Check sheet for the modelled part. Datum: model origin and axes. Units: mm. A direction names the side the tool comes from. Give positions to 0.01 mm unless a question says otherwise; leave off trailing zeros. Write each loop counter-clockwise with the first axis right and the second up, starting at its lowest first coordinate (ties: lowest second). Pieces come first, ordered by that corner, then holes. Notation, with made-up numbers: (-5.75, 47.25) -> (15.25, 47.25) arc R26 cw to (15.25, 74.25) -> close; hole circle Ø1 at (62, -2). An arc over 180 degrees is marked (long way). Write each question's results on one line, items separated by ' | '. Start each with the question number.
```python
from build123d import *

# Parameters (mm, degrees)
F0_W     = 74.9129392207
F0_H     = 89.2662387341
F0_H_2   = 11.6326007992
F1_DEPTH = 25.4
F3_DEPTH = 38.1
F4_W     = 74.9129392207
F4_H     = 18.2247254997
F5_DEPTH = 76.2
F7_DEPTH = 25.4
F8_W     = 15.1206124574
F8_H     = 39.1616150737
F9_DEPTH = 38.1


with BuildPart() as f1:
    # F0 (on Front) → F1 (new body)
    with BuildSketch(Plane.XZ):
        with Locations((-0.0017788261, 17.1041050926)):
            Rectangle(F0_W, F0_H)
        with Locations((-0.0017788261, -33.3453146741)):
            Rectangle(F0_W, F0_H_2)
    extrude(amount=F1_DEPTH)

    # F2 (on face) → F3 (cut, symmetric)
    with BuildSketch(Plane.XZ.offset(25.4)):
        with BuildLine():
            Line((8.0494598543, 36.3066755235), (8.2423314452, 36.3066755235))
            Line((8.2423314452, 36.3066755235), (8.2423314452, 87.1677733958))
            Line((8.2423314452, 87.1677733958), (-8.2423314452, 87.1677733958))
            Line((-8.2423314452, 87.1677733958), (-8.2423314452, 36.3066755235))
            Line((-8.2423314452, 36.3066755235), (-8.0494598543, 36.3066755235))
            ThreePointArc((-8.0494598543, 36.3066755235), (0, 44.3561353778), (8.0494598543, 36.3066755235))
        make_face()
        with BuildLine():
            ThreePointArc((-8.0494598543, 36.3066755235), (0, 28.2572156693), (8.0494598543, 36.3066755235))
            Line((8.0494598543, 36.3066755235), (-8.0494598543, 36.3066755235))
        make_face()
        with BuildLine():
            Line((-8.0494598543, 36.3066755235), (8.0494598543, 36.3066755235))
            ThreePointArc((8.0494598543, 36.3066755235), (0, 44.3561353778), (-8.0494598543, 36.3066755235))
        make_face()
    extrude(amount=F3_DEPTH, both=True, mode=Mode.SUBTRACT)

    # F4 (on face) → F5 (join)
    with BuildSketch(Plane.XZ.offset(25.4)):
        with Locations((-0.0017788261, -30.0492523238)):
            Rectangle(F4_W, F4_H)
    extrude(amount=F5_DEPTH)

    # F6 (on face) → F7 (cut)
    with BuildSketch(Plane.XY.offset(-20.9368895739)):
        with BuildLine():
            ThreePointArc((2.131e-07, -101.6), (-24.3546974871, -92.7994660414), (-37.4582484365, -70.4634491506))
            Line((-37.4582484365, -70.4634491506), (-37.4582484365, -101.6))
            Line((-37.4582484365, -101.6), (2.131e-07, -101.6))
        make_face()
        with BuildLine():
            ThreePointArc((37.4546907842, -70.4825595779), (24.3472225116, -92.8056778794), (2.131e-07, -101.6))
            Line((2.131e-07, -101.6), (37.4546907842, -101.6))
            Line((37.4546907842, -101.6), (37.4546907842, -70.4825595779))
        make_face()
    extrude(amount=-F7_DEPTH, mode=Mode.SUBTRACT)

    # F8 (on face) → F9 (cut)
    with BuildSketch(Plane(origin=(0, 0, 0), x_dir=(-1, 0, 0), z_dir=(0, 1, 0))):
        with Locations((-29.8943845555, -19.5808075368)):
            Rectangle(F8_W, F8_H)
    extrude(amount=-F9_DEPTH, mode=Mode.SUBTRACT)


solid = f1.part
```
Item 1: Thickness scan on probe 1 along X at (y, z) = (-20.5, 40.5); probe 2 along Z at (x, y) = (24, -73); probe 3 along Y at (x, z) = (16.5, 10). Record the ranges inside material, lowest first. Write a range as from..to.
Item 2: Depth check by flat-ended pin: pin 1 Ø4.5 at (x, y) = (31, -18) entering from -Z; pin 2 Ø16.5 at (x, z) = (31.5, -27.5) entering from +Y; pin 3 Ø19 at (y, z) = (-16, -14) entering from +X. Enter the tip coordinate at first touch or a pass-through.
Item 3: Set-up check for faces 4 (the flat face through (8.242, -13, 49)), 5 (the flat face through (30, -13, 0)), 6 (the flat face through (-1, -63, -20.937)): record each of +Z, -Z, +X, -X, +Y, -Y from which the full face is reachable in a straight line by a thin tool's end or side.
Item 4: Mould release check, pull along X, two halves, no side actions. Record for faces 1 (the flat face through (37.455, -13, 30)), 2 (the cylindrical face through (-0.18, -12.88, 28.26)), 3 (the flat face through (-23, -13, 61.737)): pulls with the +X half, pulls with the -X half, needs draft (parallel to the pull), parting line crosses it, or undercut.
Item 5: Section check D-D on z = -13. Record the boundary of the cut face in (x, y), then the cut area to 3 significant figures.
Item 6: Section check C-C on x = 0. Record the boundary of the cut face in (y, z), then the cut area to 3 significant figures.
Item 7: Section check B-B on y = -20.5. Record the boundary of the cut face in (x, z).
Item 8: Section check A-A on x = 30. Record the boundary of the cut face in (y, z).
Check sheet entries:
1) probe 1: x = -37.46..-8.24, 8.24..37.45 | probe 2: z = -39.16..-20.94 | probe 3: y = -25.4..0
2) pin 1: stops at z = 0 | pin 2: stops at y = -38.1 | pin 3: stops at x = 22.33
3) face 4: +Z, +Y, -Y | face 5: -Z, +X, +Y, -Y | face 6: +Z, +X, -X, -Y
4) face 1: pulls with the +X half | face 2: undercut | face 3: needs draft
5) outline: (-37.46, -25.4) -> (22.33, -25.4) -> (22.33, 0) -> (-37.46, 0) -> close | area: 1,520 mm^2
6) outline: (-101.6, -39.16) -> (0, -39.16) -> (0, 28.26) -> (-25.4, 28.26) -> (-25.4, -20.94) -> (-101.6, -20.94) -> close | area: 3,100 mm^2
7) outline: (-37.46, -39.16) -> (22.33, -39.16) -> (22.33, 0) -> (37.45, 0) -> (37.45, 61.74) -> (8.24, 61.74) -> (8.24, 36.31) -> (8.05, 36.31) arc R8.05 cw to (-8.05, 36.31) -> (-8.24, 36.31) -> (-8.24, 61.74) -> (-37.46, 61.74) -> close
8) outline: (-86.99, -39.16) -> (-38.1, -39.16) -> (-38.1, -20.94) -> (-86.99, -20.94) -> close; (-25.4, 0) -> (0, 0) -> (0, 61.74) -> (-25.4, 61.74) -> close
